CAD build for the part. Positions are in the model's coordinates, mm. A direction names the side the tool comes from. Give positions to 0.01 mm unless a question says otherwise; leave off trailing zeros. Order: outer loops, then holes, each group sorted by start corner. A loop starts at its lowest first (then second) coordinate and runs counter-clockwise, first axis right, second up.
Item 1: Band-saw the part on D-D on x = 19. Give the cut face in (y, z), plus the area to 3 significant figures.
Item 2: Band-saw the part on C-C on y = 17.5. Give the cut face in (x, z).
Item 3: Band-saw the part on B-B on x = 3. Give the cut face in (y, z).
Item 4: Which spindle directions (+Z, -Z, +X, -X, +Y, -Y) get a long thin tool onto all of the face, cutting with end or side? Do faces 1 (the cylindrical face through (5, 6, 3)), 2 (the flat face through (33.75, 25, 3)), 3 (the flat face through (49, 2, 3)), 4 (the flat face through (4, 6, 1)), 5 (the cylindrical face through (8.673, 15.668, 2.958)). Say none if no direction does.
Item 5: Band-saw the part on A-A on y = 5.5. Give the cut face in (x, z), plus the area to 3 significant figures.
Item 6: Two-plate mould, pull along X, no slides. Class faces 6 (the cylindrical face through (40.168, 15.827, 2.958)), 7 (the flat face through (48.64, 1.5, 2.29)), 8 (the flat face through (15.25, 26, 3)): released by +X, released by -X, zero draft, split by the parting line, or undercut.
Item 7: Flat gauge pins, fed straight in: P1, Ø1.2, axis at x = 47, z = 3, coming from the +Y side; P2, Ø0.6, axis at y = 5, z = 0.5, coming from the -X side; P3, Ø0.8, axis at x = 32.5, z = 4, coming from the -Y side; P4, Ø2, axis at y = 6, z = 1, coming from the +X side. Where does each tip first touch, or does it go through?
Item 8: Wall check: L1, parallel to X at y = 4, z = 1.5; L2, parallel to Y at x = 20.5, z = 1.5. Give the ranges that are in metal, low to high.
```python
from build123d import *

# Parameters (mm, degrees)
EXTRUDE_1_DEPTH          = 6
CUT_EXTRUDE_1_DEPTH      = 10
CUT_EXTRUDE_1_DEPTH_BACK = 10
SKETCH_2_R               = 2
CUT_EXTRUDE_START        = -10
CUT_EXTRUDE_2_DEPTH      = 10


with BuildPart() as part:
    # 스케치1 → 보스-돌출1 (new body)
    with BuildSketch(Plane.XY):
        with BuildLine():
            Line((31.75, 18.5), (33, 18.5))
            ThreePointArc((33, 18.5), (40.071067812, 15.571067812), (43, 8.5))
            Line((43, 8.5), (43, 1.5))
            Line((43, 1.5), (49, 1.5))
            Line((49, 1.5), (49, 3))
            Line((49, 3), (45, 3))
            Line((45, 3), (45, 8.5))
            ThreePointArc((45, 8.5), (41.746427842, 16.715838363), (33.75, 20.476539567))
            Line((33.75, 20.476539567), (33.75, 30.5))
            Line((33.75, 30.5), (15.25, 30.5))
            Line((15.25, 30.5), (15.25, 20.476539567))
            ThreePointArc((15.25, 20.476539567), (7.253572158, 16.715838363), (4, 8.5))
            Line((4, 8.5), (4, 3))
            Line((4, 3), (0, 3))
            Line((0, 3), (0, 1.5))
            Line((0, 1.5), (6, 1.5))
            Line((6, 1.5), (6, 8.5))
            ThreePointArc((6, 8.5), (8.928932188, 15.571067812), (16, 18.5))
            Line((16, 18.5), (17.25, 18.5))
            Line((17.25, 18.5), (17.25, 28.5))
            Line((17.25, 28.5), (31.75, 28.5))
            Line((31.75, 28.5), (31.75, 18.5))
        make_face()
    extrude(amount=EXTRUDE_1_DEPTH)

    # 스케치2 → 컷-돌출1 (cut, two sides: drawn at the far end of the back side and taken through both)
    with BuildSketch(Plane(origin=(0, 3, 0), x_dir=(1, 0, 0), z_dir=(0, 1, 0)).offset(-CUT_EXTRUDE_1_DEPTH_BACK)):
        with BuildLine():
            ThreePointArc((45, -5.345740821), (47.405791592, -5.127498531), (48.55, -3))
            ThreePointArc((48.55, -3), (47.405791592, -0.872501469), (45, -0.654259179))
            Line((45, -0.654259179), (45, -5.345740821))
        make_face()
        with BuildLine():
            Line((45, -5.345740821), (45, -0.654259179))
            ThreePointArc((45, -0.654259179), (43.45, -3), (45, -5.345740821))
        make_face()
        with Locations(Location((3, -3, 0), (0, 0, 60))):
            Circle(SKETCH_2_R)
    extrude(amount=CUT_EXTRUDE_1_DEPTH + CUT_EXTRUDE_1_DEPTH_BACK, mode=Mode.SUBTRACT)

    # 스케치3 → 컷-돌출2 (cut)
    with BuildSketch(Plane.XY.offset(6).offset(CUT_EXTRUDE_START)):
        with BuildLine():
            Line((5.75, 1.5), (5.75, 8.5))
            ThreePointArc((5.75, 8.5), (8.752155493, 15.747844507), (16, 18.75))
            Line((16, 18.75), (17, 18.75))
            Line((17, 18.75), (17, 28.75))
            Line((17, 28.75), (32, 28.75))
            Line((32, 28.75), (32, 18.75))
            Line((32, 18.75), (33, 18.75))
            ThreePointArc((33, 18.75), (40.247844507, 15.747844507), (43.25, 8.5))
            Line((43.25, 8.5), (43.25, 1.5))
            Line((43.25, 1.5), (43, 1.5))
            Line((43, 1.5), (43, 8.5))
            ThreePointArc((43, 8.5), (40.071067812, 15.571067812), (33, 18.5))
            Line((33, 18.5), (31.75, 18.5))
            Line((31.75, 18.5), (31.75, 28.5))
            Line((31.75, 28.5), (17.25, 28.5))
            Line((17.25, 28.5), (17.25, 18.5))
            Line((17.25, 18.5), (16, 18.5))
            ThreePointArc((16, 18.5), (8.928932188, 15.571067812), (6, 8.5))
            Line((6, 8.5), (6, 1.5))
            Line((6, 1.5), (5.75, 1.5))
        make_face()
    extrude(amount=CUT_EXTRUDE_2_DEPTH, mode=Mode.SUBTRACT)


solid = part.part
```
The answers:
1. outline: (28.75, 0) - (30.5, 0) - (30.5, 6) - (28.75, 6) - close
1. area: 10.5 mm2
2. outline: (8.06, 0) - (11.09, 0) - (11.09, 6) - (8.06, 6) - close; (37.91, 0) - (40.94, 0) - (40.94, 6) - (37.91, 6) - close
3. outline: (1.5, 0) - (3, 0) - (3, 1) - (1.5, 1) - close; (1.5, 5) - (3, 5) - (3, 6) - (1.5, 6) - close
4. face 1: -Y
4. face 2: +Z, -Z, +X, +Y
4. face 3: +Z, -Z, +X, +Y, -Y
4. face 4: +Z, -Z, -X, +Y
4. face 5: +Z, -Z, -Y
5. outline: (4, 0) - (5.75, 0) - (5.75, 6) - (4, 6) - (4, 4.73) arc R2 cw to (4, 1.27) - close; (43.25, 0) - (45, 0) - (45, 0.65) arc R2.55 cw to (45, 5.35) - (45, 6) - (43.25, 6) - close
5. area: 13.3 mm2
6. face 6: undercut
6. face 7: zero draft
6. face 8: released by -X
7. P1: passes through
7. P2: stops at x = 4
7. P3: stops at y = 18.75
7. P4: stops at x = 45
8. L1: x = 4.32 to 5.75, 43.25 to 43.94
8. L2: y = 28.75 to 30.5
